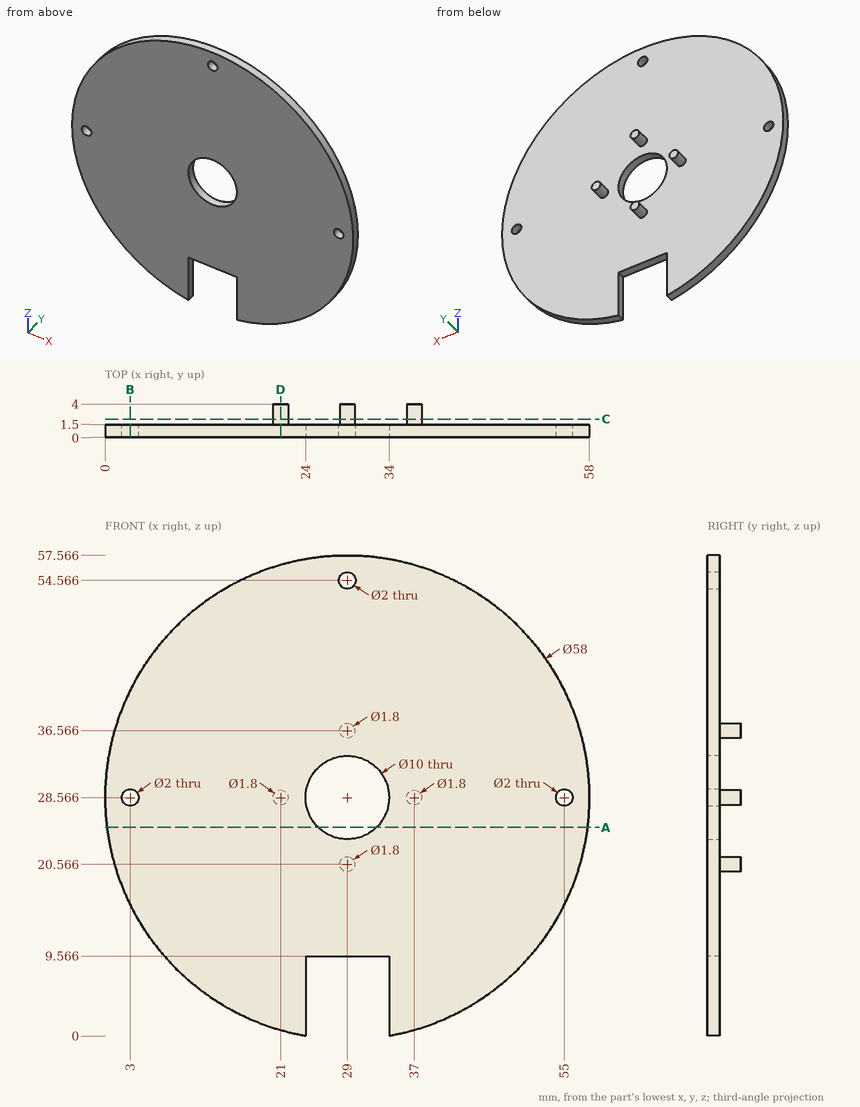
The figure shows three views and two pictorial views of one solid part (mm, origin at its lowest corner). Answer the questions. Give positions to 0.01 mm unless a question says otherwise; leave off trailing zeros. Loops run counter-clockwise (first coordinate to the right, second up) from the corner with the lowest first, then second, coordinate; pieces in that order, holes last. Notation, with made-up numbers: (16, -23) -> (63, -23) arc R15 cw to (63, -19) -> close; hole circle Ø2 at (66, -38.75). An arc over 180 degrees is marked (long way). Use a Markdown table: item, result. Add a question column.
1. Find the intervals of material crossed by probe 1 along X at (y, z) = (3.2, 28.5); probe 2 along Y at (x, z) = (37, 21); probe 3 along Z at (x, y) = (29.5, 3.85) (1 decimal), in increasing order.
2. Flat-ended cylindrical pins translate along their axes: pin 1 Ø10 at (x, z) = (19.5, 48) entering from +Y; pin 2 Ø1.2 at (y, z) = (1, 5) entering from -X; pin 3 Ø1.2 at (x, y) = (31.5, 1) entering from -Z. Find the tip coordinate at first contact, or state that the pin passes through.
3. Section A-A on z = 25 is taken. Determine the outline of the cut face in (x, y) (1 decimal).
4. Section C-C on y = 2.2 is taken. Determine the outline of the cut face in (x, z), and give its area (3 significant figures).
5. Section B-B on x = 3 is taken. Determine the outline of the cut face in (y, z).
6. Section D-D on x = 21 is taken. Determine the outline of the cut face in (y, z).
Results below:
| question | item | result |
|---|---|---|
| 1 | probe 1 | x = 20.1 to 21.9, 36.1 to 37.9 |
| 1 | probe 2 | y = 0 to 1.5 |
| 1 | probe 3 | z = 19.8 to 21.3, 35.8 to 37.3 |
| 2 | pin 1 | stops at y = 1.5 |
| 2 | pin 2 | stops at x = 11.29 |
| 2 | pin 3 | stops at z = 9.57 |
| 3 | outline | (0.2, 0) -> (25.5, 0) -> (25.5, 1.5) -> (0.2, 1.5) -> close; (32.5, 0) -> (57.8, 0) -> (57.8, 1.5) -> (32.5, 1.5) -> close |
| 4 | outline | circle Ø1.8 at (21, 28.57); circle Ø1.8 at (29, 20.57); circle Ø1.8 at (29, 36.57); circle Ø1.8 at (37, 28.57) |
| 4 | area | 10.2 mm^2 |
| 5 | outline | (0, 15.72) -> (1.5, 15.72) -> (1.5, 27.57) -> (0, 27.57) -> close; (0, 29.57) -> (1.5, 29.57) -> (1.5, 41.41) -> (0, 41.41) -> close |
| 6 | outline | (0, 0.69) -> (1.5, 0.69) -> (1.5, 27.67) -> (4, 27.67) -> (4, 29.47) -> (1.5, 29.47) -> (1.5, 56.44) -> (0, 56.44) -> close |
